Could you check a few things on this model? Use its own coordinates, in mm. Face numbers are marked on the shaded views. A direction names the side the tool comes from. Coordinates: 2 decimals unless noted, no trailing zeros. Order: outer loops, then holes, each group sorted by start corner. A loop starts at its lowest first (then second) coordinate and runs counter-clockwise, first axis right, second up. Notation, with made-up numbers: M 40,53.25 L 66,53.25 A24 cw 66,79.25 Z; hole C -27.75,25 d5. An arc over 180 degrees is marked long. Put each result on its own line as item: value. Start each with the question number.
Autodesk Inventor part; units mm, degrees
ref_plane "Work Plane1" through (1.525, 0, 0) normal (0, 0, 1) x (1, 0, 0)
ref_plane "YZ Plane" through (0, 0, 0) normal (1, 0, 0) x (0, 1, 0)
ref_plane "XZ Plane" through (0, 0, 0) normal (0, 1, 0) x (-1, 0, 0)
sketch "Sketch1" plane through (0, 0, 0) normal (0, 0, 1) x (1, 0, 0)
  line L0 (0, 7.1374) -> (0, 4.9276)
  line L1 (25.4, 4.7625) -> (152.4, 4.7625)
  line L2 (152.4, 4.7625) -> (152.4, 0)
  line L3 (152.4, 0) -> (-0.0001, 0)
  line L4 (-30.4801, 0) -> (182.88, 0)
  line L5 (-0.0001, 0) -> (-0.0001, 7.1374)
  line L6 (-0.0001, 7.1374) -> (0, 7.1374)
  line L7 (25.4, 4.7625) -> (21.4311, 4.9276)
  line L8 (21.4311, 4.9276) -> (0, 4.9276)
  line L9 (0, -1.4275) -> (0, 8.5649)
  dimension "d0" = 152.4
  dimension "d1" = 127
revolve "Body" add sketch "Sketch1" angle 360 about axis through (152.4, 0, 0) along (-1, 0, 0)
sketch "Sketch2" plane through (-0.0001, 0, 0) normal (-1, 0, 0) x (0, 0, 1)
  line L0 (0, 8.2416) -> (7.1374, 4.1208)
  line L1 (7.1374, 4.1208) -> (7.1374, -4.1208)
  line L2 (7.1374, -4.1208) -> (0, -8.2416)
  line L3 (0, -8.2416) -> (-7.1374, -4.1208)
  line L4 (-7.1374, -4.1208) -> (-7.1374, 4.1208)
  line L5 (-7.1374, 4.1208) -> (0, 8.2416)
  point P0 (0, 0)
  point P1 (0, 0)
  dimension "d11" = 14.2748
extrude "Head" add sketch "Sketch2" along normal blind 6.8072
sketch "Sketch4" plane through (0, 0, 0) normal (0, 0, 1) x (1, 0, 0)
  line L0 (-6.8073, 7.1374) -> (-6.8073, 8.2416)
  line L1 (-6.8073, 8.2416) -> (-6.1698, 8.2416)
  line L2 (-6.1698, 8.2416) -> (-6.8073, 7.1374)
  line L3 (-8.1687, 0) -> (1.3613, 0)
  line L4 (-0.0001, 8.2416) -> (-6.8073, 8.2416)
  line L5 (-6.8073, 4.1208) -> (-6.8073, 8.2416)
  dimension "d5" = 30
  dimension "d19" = 14.2748
revolve "Chamfer1" cut sketch "Sketch4" angle 360 about axis through (-10, 0, 0) along (1, 0, 0)
thread "Thread"
chamfer "Chamfer2" distance 0.9739 distance2 0.9447 1 edges at (152.4, -4.7625, 0) measured on face at (152.4, -0.1914, 1.3928)
ref_plane "Work Plane1" through (1.525, 0, 0) normal (0, 0, 1) x (1, 0, 0)
fillet "Fillet2" radius 0.762 1 edges at (0, -4.9276, 0)
equation "\"d63\" = R"
equation "\"d11\" = SW"
equation "\"d3\" = KOH - SD"
equation "\"d15\" = GEL"
equation "\"d6\" = -0.5 * SPD + 0.5 * GD"
equation "\"d5\" = ANG1"
equation "\"d19\" = SW0"
equation "\"NLG\" = 190.5"
equation "\"GD\" = NND"
equation "\"BDM\" = 9.8552"
equation "\"KOH\" = 6.8072"
equation "\"GEL\" = 31.75"
equation "\"SW\" = 14.2748"
equation "\"SW0\" = SW"
equation "\"SPD\" = GD1"
equation "\"SD2\" = SW"
equation "\"SD\" = 0"
equation "\"ANG1\" = 30deg"
equation "\"GAL\" = 3.96875"
equation "\"GUL\" = 0.238 * GAL"
equation "\"R\" = 0.762"
equation "\"d62\" = -NLG - SD + GUL"
equation "\"GD1\" = 7.5773"
equation "\"THREADDIA\" = 9.525"
equation "\"TOA\" = 30deg"
equation "\"NND\" = 9.525"
equation "\"E0\" = 1.155 * SW"
properties part number "am-1055" material "Steel, Mild"
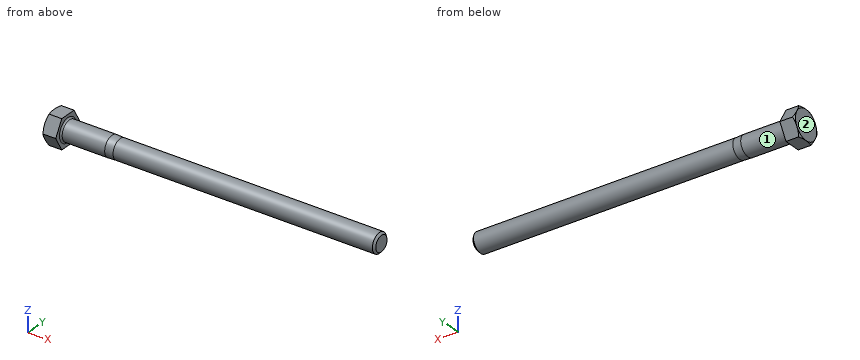
Item 1: For the marked faces 1 and 2, which set-ups out of +Z, -Z, +X, -X, +Y, -Y let a thin tool reach every point of the face, with its end or its side?
Item 2: For pin 1 Ø4 at (x, z) = (73, 1) entering from +Y; pin 2 Ø8 at (x, y) = (67.5, -3) entering from +Z; pin 3 Ø3 at (x, y) = (53, -2) entering from -Z; pin 4 Ø1 at (x, y) = (110.5, -6) entering from +Z, each with a flat end and sliding along its axis, tell me the tip position at first contact or that it passes through.
Item 3: If we section it at B-B on x = 5: Write out the boundary of the cut face in (y, z).
Item 4: I need wall thicknesses on probe 1 along X at (y, z) = (2, -3.25); probe 2 along X at (y, z) = (0.75, -5.75); probe 3 along Z at (x, y) = (113.5, -0.25). Which ranges of each line are inside material? Lowest first, please.
Item 5: If we section it at A-A on x = 139.5: Write out the boundary of the cut face in (y, z) (1 decimal).
Geometry check:
1. face 1: +X
1. face 2: +Z, -Z, -X, +Y, -Y
2. pin 1: stops at y = 4.76
2. pin 2: stops at z = 4.76
2. pin 3: stops at z = -4.74
2. pin 4: passes through
3. outline: C 0,0 d9.86
4. probe 1: x = -6.81 to 152.37
4. probe 2: x = -6.81 to 0
4. probe 3: z = -4.76 to 4.76
5. outline: C 0,0 d9.5
